from build123d import *

# Parameters (mm, degrees)
F0_R          = 4.826
F1_DEPTH      = 44.45
F1_DEPTH_BACK = 44.45
F3_DEPTH      = 76.2
F3_DEPTH_BACK = 76.2
F4_R          = 3.175
F5_DEPTH      = 25.4


with BuildPart() as f1:
    # F0 (on Right) → F1 (new body, two sides)
    with BuildSketch(Plane.YZ) as f1_sk:
        with BuildLine():
            Line((-58.42, -10.16), (58.42, -10.16))
            ThreePointArc((58.42, -10.16), (63.808154, -7.928154), (66.04, -2.54))
            Line((66.04, -2.54), (66.04, 59.69))
            Line((66.04, 59.69), (-66.04, 59.69))
            Line((-66.04, 59.69), (-66.04, -2.54))
            ThreePointArc((-66.04, -2.54), (-63.808154, -7.928154), (-58.42, -10.16))
        make_face()
        with Locations((-54.356, 0)):
            Circle(F0_R, mode=Mode.SUBTRACT)
        with Locations((54.356, 0)):
            Circle(F0_R, mode=Mode.SUBTRACT)
    extrude(amount=F1_DEPTH)
    extrude(f1_sk.sketch, amount=-F1_DEPTH_BACK)

    # F2 (on Front) → F3 (cut, two sides)
    with BuildSketch(Plane.XZ) as f3_sk:
        with BuildLine():
            Line((41.275, -10.16), (41.275, -2.54))
            Line((41.275, -2.54), (41.275, 52.705))
            ThreePointArc((41.275, 52.705), (40.159077, 55.399077), (37.465, 56.515))
            Line((37.465, 56.515), (-37.465, 56.515))
            ThreePointArc((-37.465, 56.515), (-40.159077, 55.399077), (-41.275, 52.705))
            Line((-41.275, 52.705), (-41.275, -2.54))
            Line((-41.275, -2.54), (-41.275, -10.16))
            Line((-41.275, -10.16), (41.275, -10.16))
        make_face()
    extrude(amount=F3_DEPTH, mode=Mode.SUBTRACT)
    extrude(f3_sk.sketch, amount=-F3_DEPTH_BACK, mode=Mode.SUBTRACT)

    # F4 (on face) → F5 (cut)
    with BuildSketch(Plane.XY.offset(59.69)):
        with Locations((28.575, -38.1)):
            Circle(F4_R)
        with Locations((-28.575, -38.1)):
            Circle(F4_R)
        with Locations((-28.575, 38.1)):
            Circle(F4_R)
        with Locations((28.575, 38.1)):
            Circle(F4_R)
    extrude(amount=-F5_DEPTH, mode=Mode.SUBTRACT)


solid = f1.part
Could you check a few things on this model? Use its own coordinates, in mm. A direction names the side the tool comes from. Give positions to 0.01 mm unless a question says otherwise; leave off trailing zeros. Loops run counter-clockwise (first coordinate to the right, second up) from the corner with the lowest first, then second, coordinate; pieces in that order, holes last. Notation, with made-up numbers: (29.25, 46) -> (57.25, 46) arc R25 ccw to (57.25, 63) -> close; hole circle Ø11 at (59, -17.75). An arc over 180 degrees is marked (long way). Return JSON: item names as keys, results as strings.
Item 1: If we section it at B-B on y = 38.1: List the corners of the cut face in (x, z) for me (3 decimals).
Geometry results:
{"outline": "(-44.45, -10.16) -> (-41.275, -10.16) -> (-41.275, 52.705) arc R3.81 cw to (-37.465, 56.515) -> (-31.75, 56.515) -> (-31.75, 59.69) -> (-44.45, 59.69) -> close; (-25.4, 56.515) -> (25.4, 56.515) -> (25.4, 59.69) -> (-25.4, 59.69) -> close; (31.75, 56.515) -> (37.465, 56.515) arc R3.81 cw to (41.275, 52.705) -> (41.275, -10.16) -> (44.45, -10.16) -> (44.45, 59.69) -> (31.75, 59.69) -> close"}
Item 2: If we section it at A-A on z = 26: List the corners of the cut face in (x, y) for me (3 decimals), plus the area to 3 significant figures.
Geometry results:
{"outline": "(-44.45, -66.04) -> (-41.275, -66.04) -> (-41.275, 66.04) -> (-44.45, 66.04) -> close; (41.275, -66.04) -> (44.45, -66.04) -> (44.45, 66.04) -> (41.275, 66.04) -> close", "area": "839 mm²"}
Item 3: I'm going to push flat-ended pins straight in: pin 1 (7.5 mm diameter, centred on x = -28.575, y = 38.1, fed in from +Z); pin 2 (5 mm diameter, centred on x = 28.575, y = -38.1, fed in from +Z); pin 3 (1.5 mm diameter, centred on x = -10, y = 6.5, fed in from -Z) (3 decimals). Where does each tip first touch, or does it pass through?
Geometry results:
{"pin 1": "stops at z = 59.69", "pin 2": "passes through", "pin 3": "stops at z = 56.515"}
Item 4: I need wall thicknesses on L1, parallel to Y at x = 42.7, z = 0; L2, parallel to X at y = -27, z = 5 (3 decimals); L3, parallel to Z at x = -26, y = 57.5 (3 decimals). Which ranges of each line are inside material? Lowest first, please. Write a range as from..to.
Geometry results:
{"L1": "y = -66.04..-59.18, -49.53..49.53, 59.18..66.04", "L2": "x = -44.45..-41.275, 41.275..44.45", "L3": "z = 56.515..59.69"}
Item 5: If we section it at C-C on z = 0: List the corners of the cut face in (x, y) for me (3 decimals), plus the area to 3 significant figures.
Geometry results:
{"outline": "(-44.45, -66.04) -> (-41.275, -66.04) -> (-41.275, -59.182) -> (-44.45, -59.182) -> close; (-44.45, -49.53) -> (-41.275, -49.53) -> (-41.275, 49.53) -> (-44.45, 49.53) -> close; (-44.45, 59.182) -> (-41.275, 59.182) -> (-41.275, 66.04) -> (-44.45, 66.04) -> close; (41.275, -66.04) -> (44.45, -66.04) -> (44.45, -59.182) -> (41.275, -59.182) -> close; (41.275, -49.53) -> (44.45, -49.53) -> (44.45, 49.53) -> (41.275, 49.53) -> close; (41.275, 59.182) -> (44.45, 59.182) -> (44.45, 66.04) -> (41.275, 66.04) -> close", "area": "716 mm²"}
Item 6: Which directions (+Z, -Z, +X, -X, +Y, -Y) give clear straight access to the entire face, cutting with the end or side of a thin tool? Please do faces 1 (the flat face through (-44.45, -1, 25)), 2 (the cylindrical face through (-40.13, 0.92, 55.43)).
Geometry results:
{"face 1": "+Z, -Z, -X, +Y, -Y", "face 2": "-Z, +Y, -Y"}
Item 7: We'd pull the mould along Y, two halves only. Please class faces 3 (the cylindrical face through (-42.88, 58.96, 1.45)), 4 (the cylindrical face through (26.055, 36.168, 58.125)), 5 (the cylindrical face through (42.885, -63.867, -7.869)), 6 (the flat face through (0, 66.04, 58)): +Y half, -Y half, draft (parallel to the pull), parting line (faces both ways), or undercut.
Geometry results:
{"face 3": "undercut", "face 4": "undercut", "face 5": "-Y half", "face 6": "+Y half"}
Item 8: If we section it at D-D on x = -14: List the corners of the cut face in (y, z) for me (3 decimals).
Geometry results:
{"outline": "(-66.04, 56.515) -> (66.04, 56.515) -> (66.04, 59.69) -> (-66.04, 59.69) -> close"}
